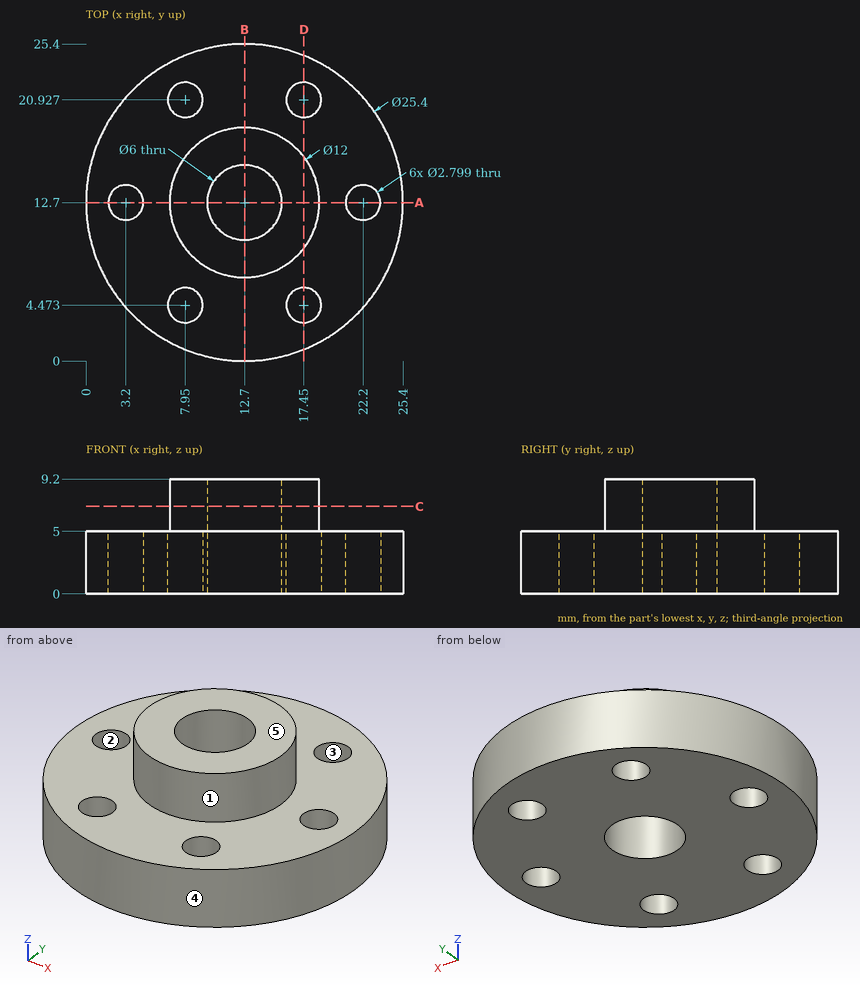
Job drawing, mm, ordinate dimensions from the low corner. One solid piece. A direction names the side the tool comes from. Coordinates: 2 decimals unless noted, no trailing zeros. Order: outer loops, then holes, each group sorted by start corner. A loop starts at its lowest first (then second) coordinate and runs counter-clockwise, first axis right, second up. Notation, with made-up numbers: (43.25, 23) - (54.25, 23) arc R24 cw to (54.25, 40) - close; hole circle Ø2 at (-29.5, 58.25). An arc over 180 degrees is marked (long way). Use CSV: the item, a comma, the result in double quotes.
Item 1: Drop flat-ended pins along their axis: P1, Ø3.5, axis at x = 7.95, y = 20.93, coming from the +Z side; P2, Ø2.5, axis at x = 17.45, y = 4.47, coming from the +Z side; P3, Ø5, axis at y = 6.5, z = 5.5, coming from the +X side. Give the stop position or say it passes through.
Solved:
P1,"stops at z = 5"
P2,"passes through"
P3,"stops at x = 24.83"
Item 2: Probe probe 1 along X at (y, z) = (20.25, 3.5) (1 decimal); probe 2 along Y at (x, z) = (12.7, 4); probe 3 along Y at (x, z) = (7.95, 2.6). List the from-to ranges inside material, lowest first.
Solved:
probe 1,"x = 2.5 to 6.7, 9.2 to 16.2, 18.7 to 22.9"
probe 2,"y = 0 to 9.7, 15.7 to 25.4"
probe 3,"y = 0.92 to 3.07, 5.87 to 19.53, 22.33 to 24.48"
Item 3: Saw through at B-B on x = 12.7. Give the cut face in (y, z).
Solved:
outline,"(0, 0) - (9.7, 0) - (9.7, 9.2) - (6.7, 9.2) - (6.7, 5) - (0, 5) - close; (15.7, 0) - (25.4, 0) - (25.4, 5) - (18.7, 5) - (18.7, 9.2) - (15.7, 9.2) - close"
Item 4: Saw through at A-A on y = 12.7. Give the cut face in (x, z).
Solved:
outline,"(0, 0) - (1.8, 0) - (1.8, 5) - (0, 5) - close; (4.6, 0) - (9.7, 0) - (9.7, 9.2) - (6.7, 9.2) - (6.7, 5) - (4.6, 5) - close; (15.7, 0) - (20.8, 0) - (20.8, 5) - (18.7, 5) - (18.7, 9.2) - (15.7, 9.2) - close; (23.6, 0) - (25.4, 0) - (25.4, 5) - (23.6, 5) - close"
Item 5: Mould opens along X. For the marked faces 3, 4 and 5 say: +X half, -X half, draft (parallel to the pull), parting line (faces both ways), or undercut.
Solved:
face 3,"undercut"
face 4,"parting line"
face 5,"draft"
Item 6: Saw through at D-D on x = 17.45. Give the cut face in (y, z).
Solved:
outline,"(0.92, 0) - (3.07, 0) - (3.07, 5) - (0.92, 5) - close; (5.87, 0) - (19.53, 0) - (19.53, 5) - (16.37, 5) - (16.37, 9.2) - (9.03, 9.2) - (9.03, 5) - (5.87, 5) - close; (22.33, 0) - (24.48, 0) - (24.48, 5) - (22.33, 5) - close"
Item 7: 3-axis set-ups, long thin cutter, end or side, ignore diameter. For the marked faces 1 and 2: which of +Z, -Z, +X, -X, +Y, -Y reach the whole face in a straight line?
Solved:
face 1,"+Z"
face 2,"+Z, -Z"
Item 8: Saw through at C-C on z = 7. Give the cut face in (x, y).
Solved:
outline,"circle Ø12 at (12.7, 12.7); hole circle Ø6 at (12.7, 12.7)"
